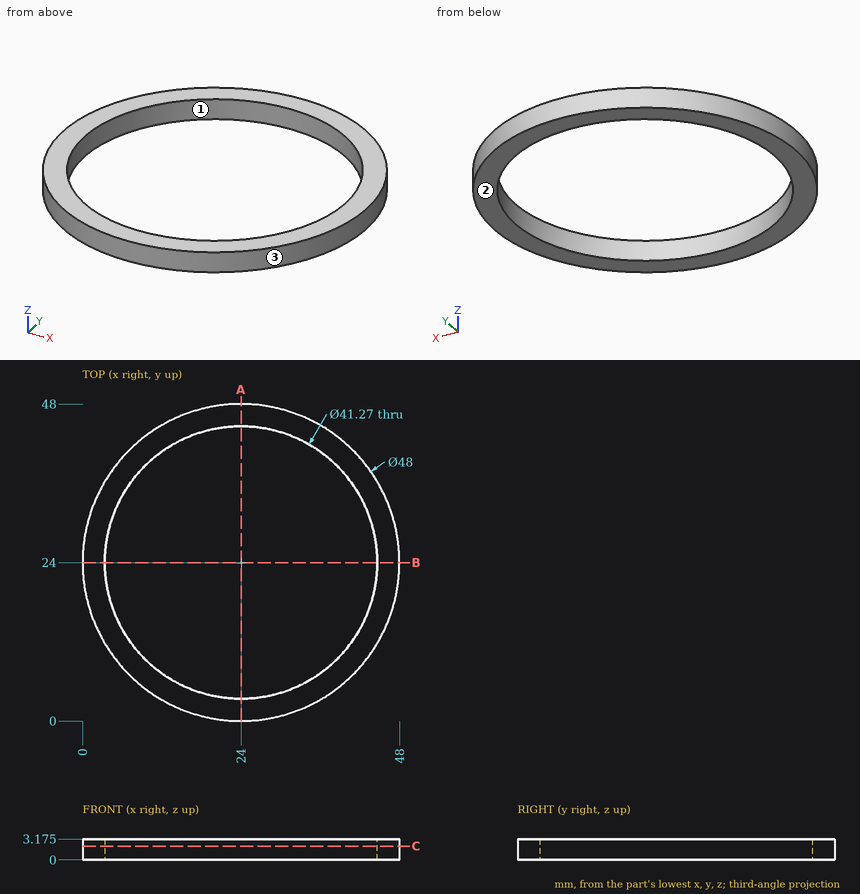
Here's the drawing with two shaded views (mm, measured from the low corner). I have some questions. Give positions to 0.01 mm unless a question says otherwise; leave off trailing zeros. Order: outer loops, then holes, each group sorted by start corner. A loop starts at its lowest first (then second) coordinate and runs counter-clockwise, first axis right, second up. Notation, with made-up numbers: (20.25, -8) -> (50.25, -8) arc R21 ccw to (50.25, 0) -> close; hole circle Ø4 at (35.5, -11.5). An arc over 180 degrees is marked (long way). Use a Markdown table: item, result. Add a question column.
Item 1: If we mould it in two halves opening along X, with no side actions, what happens to the marked faces 1, 2 and 3? For each: pulls with the +X half, pulls with the -X half, needs draft (parallel to the pull), parting line crosses it, or undercut.
Item 2: I need wall thicknesses on line 1 (Y direction, x = 24, z = 1.8) (3 decimals); line 2 (X direction, y = 24.5, z = 2.45); line 3 (Y direction, x = 17.5, z = 2.5). Which ranges of each line are inside material? Lowest first, please.
Item 3: Imagine slicing it at A-A on x = 24. Please give me the cut outline in (y, z) (3 decimals).
Item 4: Imagine slicing it at C-C on z = 2.1. Please give me the cut outline in (x, y) (3 decimals), plus the area to 3 significant figures.
Data:
| question | item | result |
|---|---|---|
| 1 | face 1 | undercut |
| 1 | face 2 | needs draft |
| 1 | face 3 | parting line crosses it |
| 2 | line 1 | y = 0 to 3.365, 44.635 to 48 |
| 2 | line 2 | x = 0.01 to 3.37, 44.63 to 47.99 |
| 2 | line 3 | y = 0.9 to 4.42, 43.58 to 47.1 |
| 3 | outline | (0, 0) -> (3.365, 0) -> (3.365, 3.175) -> (0, 3.175) -> close; (44.635, 0) -> (48, 0) -> (48, 3.175) -> (44.635, 3.175) -> close |
| 4 | outline | circle Ø48 at (24, 24); hole circle Ø41.27 at (24, 24) |
| 4 | area | 472 mm² |
